```python
from build123d import *

# Parameters (mm, degrees)
CHAMFER1_SIZE                    = 0.762
F_3_8_0_375_DIAMETER_HOLE1_D     = 9.525
F_3_8_0_375_DIAMETER_HOLE1_DEPTH = 38.1
F_3_8_0_375_DIAMETER_HOLE1_TIP   = 1.733408241
F_3_8_0_375_DIAMETER_HOLE2_D     = 1.524
F_3_8_0_375_DIAMETER_HOLE2_DEPTH = 38.1
F_3_8_0_375_DIAMETER_HOLE2_TIP   = 0.277345319
F_3_8_0_375_DIAMETER_HOLE3_D     = 9.652
F_3_8_0_375_DIAMETER_HOLE3_DEPTH = 4.826
F_3_8_0_375_DIAMETER_HOLE3_TIP   = 1.756520351
EXTRUDE1_DEPTH                   = 25.4
EXTRUDE1_DEPTH_BACK              = 25.4
SKETCH10_W                       = 9.652
SKETCH10_H                       = 2.627899037
SKETCH10_H_2                     = 6.35
CUT_EXTRUDE1_DEPTH               = 12.7


with BuildPart() as part:
    # Sketch1 → Revolve1 (revolve)
    with BuildSketch(Plane.XY):
        Polygon((0, 0), (0, 7.112), (12.7, 12.446), (25.4, 12.446), (25.4, 8.001), (26.924, 8.001), (26.924, 9.525), (50.8, 9.525), (50.8, 0), align=None)
    revolve(axis=Axis((50.8, 0, 0), (-1, 0, 0)))

    # Chamfer1
    chamfer1_edges = [part.edges().sort_by_distance(p)[0] for p in [
        (50.8, -9.525, 0),
    ]]
    chamfer(chamfer1_edges, length=CHAMFER1_SIZE)

    # 3/8 (0.375) Diameter Hole1
    with Locations(Plane(origin=(50.8, 0, 0), x_dir=(0, 0, -1), z_dir=(1, 0, 0))):
        with Locations((0, 0)):
            Hole(F_3_8_0_375_DIAMETER_HOLE1_D / 2, depth=F_3_8_0_375_DIAMETER_HOLE1_DEPTH)
            with Locations((0, 0, -(F_3_8_0_375_DIAMETER_HOLE1_DEPTH + F_3_8_0_375_DIAMETER_HOLE1_TIP / 2))):  # 140° drill point
                Cone(0, F_3_8_0_375_DIAMETER_HOLE1_D / 2, F_3_8_0_375_DIAMETER_HOLE1_TIP, mode=Mode.SUBTRACT)

    # 3/8 (0.375) Diameter Hole2
    with Locations(Plane.ZY):
        with Locations((0, 0)):
            Hole(F_3_8_0_375_DIAMETER_HOLE2_D / 2, depth=F_3_8_0_375_DIAMETER_HOLE2_DEPTH)
            with Locations((0, 0, -(F_3_8_0_375_DIAMETER_HOLE2_DEPTH + F_3_8_0_375_DIAMETER_HOLE2_TIP / 2))):  # 140° drill point
                Cone(0, F_3_8_0_375_DIAMETER_HOLE2_D / 2, F_3_8_0_375_DIAMETER_HOLE2_TIP, mode=Mode.SUBTRACT)

    # 3/8 (0.375) Diameter Hole3
    with Locations(Plane.ZY):
        with Locations((0, 0)):
            Hole(F_3_8_0_375_DIAMETER_HOLE3_D / 2, depth=F_3_8_0_375_DIAMETER_HOLE3_DEPTH)
            with Locations((0, 0, -(F_3_8_0_375_DIAMETER_HOLE3_DEPTH + F_3_8_0_375_DIAMETER_HOLE3_TIP / 2))):  # 140° drill point
                Cone(0, F_3_8_0_375_DIAMETER_HOLE3_D / 2, F_3_8_0_375_DIAMETER_HOLE3_TIP, mode=Mode.SUBTRACT)

    # Sketch10 → Extrude1 (cut, two sides: drawn at the far end of the back side and taken through both)
    with BuildSketch(Plane.XY.offset(-EXTRUDE1_DEPTH_BACK)):
        with Locations((20.574, 12.489949519)):
            Rectangle(SKETCH10_W, SKETCH10_H)
        with Locations((20.574, -14.351)):
            Rectangle(SKETCH10_W, SKETCH10_H_2)
    extrude(amount=EXTRUDE1_DEPTH + EXTRUDE1_DEPTH_BACK, mode=Mode.SUBTRACT)

    # Sketch11 → Cut-Extrude1 (cut, symmetric)
    with BuildSketch(Plane.XY):
        with BuildLine():
            Line((0, 0.9921875), (0, -0.9921875))
            Line((0, -0.9921875), (0.9921875, -0.9921875))
            ThreePointArc((0.9921875, -0.9921875), (1.984375, 0), (0.9921875, 0.9921875))
            Line((0.9921875, 0.9921875), (0, 0.9921875))
        make_face()
    extrude(amount=CUT_EXTRUDE1_DEPTH, both=True, mode=Mode.SUBTRACT)


solid = part.part
```
The listing builds one solid part. Answer for the finished solid, in the listing's coordinates (mm). A direction names the side the tool comes from. Round coordinates to 2 decimals unless told otherwise and drop trailing zeros. Loops run counter-clockwise (first coordinate to the right, second up) from the corner with the lowest first, then second, coordinate; pieces in that order, holes last. Notation, with made-up numbers: (-25.75, 45.5) - (-21.75, 45.5) arc R16 cw to (-21.75, 71.5) - close; hole circle Ø5 at (55, 52.5). An arc over 180 degrees is marked (long way). Return JSON: item names as keys, results as strings. Group by question number.
1. The mould has two halves that part along Z. Classify faces 6 (the flat face through (0.5, 0.992, 6.1)), 7 (the conical face through (3.62, 3.98, 7.66)), 8 (the cylindrical face through (31.48, -2.9, -3.78)): pulls with the +Z half, pulls with the -Z half, needs draft (parallel to the pull), parting line crosses it, or undercut.
2. Consider probe 1 along Z at (x, y) = (42, 0) (1 decimal); probe 2 along Y at (x, z) = (3.4, 0); probe 3 along Y at (x, z) = (23, -5). Determine where each line is inside the solid, lowest interval first.
3. The part is cut by section A-A on y = 0. Determine the outline of the cut face in (x, z) (1 decimal).
4. Which of the six approach directions +Z, -Z, +X, -X, +Y, -Y give full straight-line access (tool end or side, diameter ignored) to faces 1 (the flat face through (0.5, -0.992, -6.1)), 2 (the cylindrical face through (38.643, -7.559, 5.796)), 3 (the flat face through (21, -11.176, 0)), 4 (the flat face through (15.748, 12, 0)), 5 (the cylindrical face through (26.17, -1.73, 7.81))?
5. Each of these flat-tipped pins is pushed along its axis until it touches: P1, Ø0.6, axis at y = 12, z = -1.5, coming from the +X side; P2, Ø1, axis at x = 12, z = 3.5, coming from the -Y side; P3, Ø8, axis at x = 16.5, y = -7, coming from the +Z side. Where does it stop, or does it pass through?
6. The part is cut by section D-D on x = 14.5. Determine the outline of the cut face in (y, z) (1 decimal), then the cut area to 3 significant figures.
7. The part is cut by section B-B on x = 22.5. Determine the outline of the cut face in (y, z) (1 decimal).
Resolved:
{
 "1": {"face 6": "needs draft", "face 7": "parting line crosses it", "face 8": "undercut"},
 "2": {"probe 1": "z = -9.5 to -4.8, 4.8 to 9.5", "probe 2": "y = -8.54 to -4.83, 4.83 to 8.54", "probe 3": "y = -11.18 to 11.18"},
 "3": {"outline": "(2, -7.9) - (12.7, -12.4) - (25.4, -12.4) - (25.4, -8) - (26.9, -8) - (26.9, -9.5) - (50, -9.5) - (50.8, -8.8) - (50.8, -4.8) - (12.7, -4.8) - (11.2, -0.8) - (6.3, -0.8) - (4.8, -4.8) - (2, -4.8) - close; (2, 4.8) - (4.8, 4.8) - (6.3, 0.8) - (11.2, 0.8) - (12.7, 4.8) - (50.8, 4.8) - (50.8, 8.8) - (50, 9.5) - (26.9, 9.5) - (26.9, 8) - (25.4, 8) - (25.4, 12.4) - (12.7, 12.4) - (2, 7.9) - close"},
 "4": {"face 1": "+Z, -Z, -X", "face 2": "+X", "face 3": "+Z, -Z, +X, -Y", "face 4": "+Z, -Z, +X, +Y", "face 5": "none"},
 "5": {"P1": "stops at x = 15.75", "P2": "stops at y = -11.9", "P3": "stops at z = 12.08"},
 "6": {"outline": "circle Ø24.9 at (0, 0); hole circle Ø9.5 at (0, 0)", "area": "415 mm²"},
 "7": {"outline": "(-11.2, -5.5) arc R12.4 ccw to (11.2, -5.5) - (11.2, 5.5) arc R12.4 ccw to (-11.2, 5.5) - close; hole circle Ø9.5 at (0, 0)"}
}
